```python
from build123d import *

# Parameters (mm, degrees)
EXTRUDE_3_DEPTH     = 15
SKETCH_6_R          = 12.5
CUT_EXTRUDE_3_DEPTH = 100
SKETCH_7_R          = 12.5
CUT_EXTRUDE_4_DEPTH = 45


with BuildPart() as part:
    # 草图5 → 凸台-拉伸3 (new, symmetric)
    with BuildSketch(Plane.XY):
        Polygon((15, 15), (50, 15), (50, -15), (-50, -15), (-50, 15), (-15, 15), (-15, 45), (15, 45), align=None)
    extrude(amount=EXTRUDE_3_DEPTH, both=True)

    # 草图6 → 切除-拉伸3 (cut)
    with BuildSketch(Plane(origin=(50, 0, 0), x_dir=(0, 0, -1), z_dir=(1, 0, 0))):
        Circle(SKETCH_6_R)
    extrude(amount=-CUT_EXTRUDE_3_DEPTH, mode=Mode.SUBTRACT)

    # 草图7 → 切除-拉伸4 (cut)
    with BuildSketch(Plane(origin=(0, 45, 0), x_dir=(1, 0, 0), z_dir=(0, 1, 0))):
        with Locations(Location((0, 0, 0), (0, 0, 270))):
            Circle(SKETCH_7_R)
    extrude(amount=-CUT_EXTRUDE_4_DEPTH, mode=Mode.SUBTRACT)


solid = part.part
```
The model under review builds one solid part; all positions refer to its coordinate system, in mm. A direction names the side the tool comes from. Round coordinates to 2 decimals unless told otherwise and drop trailing zeros. Write each loop counter-clockwise with the first axis right and the second up, starting at its lowest first coordinate (ties: lowest second). Pieces come first, ordered by that corner, then holes. Notation, with made-up numbers: (85.25, -0.75) -> (117.25, -0.75) arc R23 cw to (117.25, 38.25) -> close; hole circle Ø9 at (-25, 5). An arc over 180 degrees is marked (long way). Use CSV: the item, a comma, the result in double quotes.
Q1. Consider section C-C (x = 14). Give the boundary of the cut face in (y, z), then the cut area to 3 significant figures.
Checks:
outline,"(-15, -15) -> (45, -15) -> (45, 15) -> (-15, 15) -> close; hole circle Ø25 at (0, 0)"
area,"1,310 mm²"
Q2. For faces 1 (the flat face through (-33, 15, 0)), 2 (the flat face through (50, 14, 0)), 3 (the cylindrical face through (-7.606, 27.815, -9.92)), 4 (the flat face through (32, 15, 0)), 5 (the flat face through (-14, 45, 0)), list the 3-axis set-ups (+Z, -Z, +X, -X, +Y, -Y) from which the entire face can be reached by the end or side of a thin tool; tool diameter is ignored.
Checks:
face 1,"+Z, -Z, -X, +Y"
face 2,"+Z, -Z, +X, +Y, -Y"
face 3,"+Y"
face 4,"+Z, -Z, +X, +Y"
face 5,"+Z, -Z, +X, -X, +Y"
Q3. Consider section A-A (z = 0). Give the boundary of the cut face in (x, y).
Checks:
outline,"(-50, -15) -> (50, -15) -> (50, -12.5) -> (-50, -12.5) -> close; (-50, 12.5) -> (-12.5, 12.5) -> (-12.5, 45) -> (-15, 45) -> (-15, 15) -> (-50, 15) -> close; (12.5, 12.5) -> (50, 12.5) -> (50, 15) -> (15, 15) -> (15, 45) -> (12.5, 45) -> close"
Q4. Consider section B-B (y = 31). Give the boundary of the cut face in (x, z).
Checks:
outline,"(-15, -15) -> (15, -15) -> (15, 15) -> (-15, 15) -> close; hole circle Ø25 at (0, 0)"
Q5. For pin 1 Ø15 at (y, z) = (32, 2.5) entering from -X; pin 2 Ø15 at (y, z) = (30.5, -0.5) entering from +X; pin 3 Ø3 at (x, z) = (-2, -1) entering from +Y; pin 4 Ø6 at (y, z) = (6.5, -5) entering from +X, all flat-tipped, find the tip position at first contact; note any pin that passes through.
Checks:
pin 1,"x = -15"
pin 2,"x = 15"
pin 3,"y = -12.25"
pin 4,"through"
Q6. To check wall thickness, follow probe 1 along X at (y, z) = (40, -0.25); probe 2 along X at (y, z) = (13.5, 0). State the ranges of each line that lie inside material, in increasing order. Write a range as [from, to].
Checks:
probe 1,"[-15, -12.5], [12.5, 15]"
probe 2,"[-50, -12.5], [12.5, 50]"
Q7. Consider section D-D (y = -9). Give the boundary of the cut face in (x, z), then the cut area to 3 significant figures.
Checks:
outline,"(-50, -15) -> (50, -15) -> (50, -8.67) -> (-50, -8.67) -> close; (-50, 8.67) -> (50, 8.67) -> (50, 15) -> (-50, 15) -> close"
area,"1,270 mm²"
Q8. Mouldability with a two-part tool opening along Z and no side actions: class faces 6 (the flat face through (1, 9, 15)), 7 (the flat face through (1, 9, -15)), 8 (the cylindrical face through (0.7, -12.203, 2.71)), 9 (the flat face through (1, -15, 0)) as released by +Z, released by -Z, zero draft, split by the parting line, or undercut.
Checks:
face 6,"released by +Z"
face 7,"released by -Z"
face 8,"undercut"
face 9,"zero draft"
